Geometry: final body of the model. Coordinates: model frame, mm. A direction names the side the tool comes from. Coordinates: 2 decimals unless noted, no trailing zeros. Loops run counter-clockwise (first coordinate to the right, second up) from the corner with the lowest first, then second, coordinate; pieces in that order, holes last. Notation, with made-up numbers: (-7, 66.25) -> (48, 66.25) arc R23 cw to (48, 92.25) -> close; hole circle Ø8 at (-32, 89). An arc over 180 degrees is marked (long way). One line per item, written item: value. Start each with the question number.
Item 1: Contact query for flat-ended pins moving along their axis: pin 1 Ø5 at (x, y) = (-22, -31.5) entering from +Z; pin 2 Ø5 at (x, z) = (-63, 3.5) entering from -Y; pin 3 Ø11.5 at (x, z) = (-56.5, 30.5) entering from -Y; pin 4 Ø8.5 at (x, y) = (-47.5, -6.5) entering from +Z. Output: stop coordinate, or through.
Item 2: Mould query, pull axis X, two halves, no side actions, for faces 1 (the flat face through (0, -38, 24)), 2 (the flat face through (-11.313, -38, 29)), 3 (the flat face through (-91, -76.2, 24)). Classes: +X half, -X half, draft (parallel to the pull), parting line (faces both ways), or undercut.
Item 3: Ray query, probe 1 along X at (y, z) = (-60, 45.5); probe 2 along Y at (x, z) = (-90, 24.5); probe 3 along Y at (x, z) = (-21, 45). Return the intervals inside material, ascending. Write a range as from..to.
Item 4: Set-up query: faces 4 (the cylindrical face through (-10.787, -73.222, 43.681)), 5 (the flat face through (-51, -6, 23.301)), 6 (the flat face through (-53, -37, 9.625)), 7 (the flat face through (-51, -63.792, 5)). Return all of +Z, -Z, +X, -X, +Y, -Y with unobstructed straight access to the full face (end or side cutting, diameter ignored); none if empty.
Item 5: Section query D-D on y = -68. Return loops of the section in (x, z).
Item 6: Section query C-C on y = -44. Return loops of the section in (x, z).
Item 7: Section query A-A on z = 37. Return loops of the section in (x, y).
Item 8: Section query B-B on x = -60. Return loops of the section in (y, z).
from build123d import *

# Parameters (mm, degrees)
F0_W      = 101.346001029
F0_H      = 47.725263983
F1_DEPTH  = 76.2
F2_W      = 81.5831655636
F2_H      = 52.9085965827
F3_DEPTH  = 38.1
F4_W      = 58.673998341
F4_H      = 24.4241077453
F5_DEPTH  = 76.2
F6_W      = 58.673998341
F6_H      = 12.4078532577
F7_DEPTH  = 50.8
F8_R      = 3.5544652988
F9_DEPTH  = 127
F10_R     = 3.7666020305
F11_DEPTH = 127


with BuildPart() as f1:
    # F0 (on Front) → F1 (new body)
    with BuildSketch(Plane.XZ):
        with Locations((-50.6730005145, 23.8626319915)):
            Rectangle(F0_W, F0_H)
    extrude(amount=F1_DEPTH)

    # F2 (on face) → F3 (cut)
    with BuildSketch(Plane.XY.offset(47.725263983)):
        with Locations((-52.104968112, -37.337848451)):
            Rectangle(F2_W, F2_H)
    extrude(amount=-F3_DEPTH, mode=Mode.SUBTRACT)

    # F4 (on face) → F5 (cut)
    with BuildSketch(Plane.XZ.offset(76.2)):
        with Locations((-50.6128417328, 35.5132101104)):
            Rectangle(F4_W, F4_H)
    extrude(amount=-F5_DEPTH, mode=Mode.SUBTRACT)

    # F6 (on face) → F7 (cut)
    with BuildSketch(Plane.XY.offset(23.3011562377)):
        with Locations((-50.6128417328, -69.9960733712)):
            Rectangle(F6_W, F6_H)
    extrude(amount=-F7_DEPTH, mode=Mode.SUBTRACT)

    # F8 (on face) → F9 (cut)
    with BuildSketch(Plane(origin=(-101.346001029, 0, 0), x_dir=(0, -1, 0), z_dir=(-1, 0, 0))):
        with Locations((68.0850967765, 9.1249775141)):
            Circle(F8_R)
    extrude(amount=-F9_DEPTH, mode=Mode.SUBTRACT)

    # F10 (on face) → F11 (cut)
    with BuildSketch(Plane(origin=(-101.346001029, 0, 0), x_dir=(0, -1, 0), z_dir=(-1, 0, 0))):
        with Locations((69.6296393871, 42.5492078066)):
            Circle(F10_R)
    extrude(amount=-F11_DEPTH, mode=Mode.SUBTRACT)


solid = f1.part
Reply:
1. pin 1: stops at z = 9.63
1. pin 2: stops at y = -63.79
1. pin 3: passes through
1. pin 4: stops at z = 23.3
2. face 1: +X half
2. face 2: undercut
2. face 3: draft
3. probe 1: x = -101.35..-92.9, -11.31..0
3. probe 2: y = -76.2..-63.79, -10.88..0
3. probe 3: y = -76.2..-72.49, -66.77..-63.79, -10.88..0
4. face 4: +X, -X
4. face 5: +Z, +Y, -Y
4. face 6: +Z
4. face 7: +Z, -Z, -Y
5. outline: (-101.35, 0) -> (-79.95, 0) -> (-79.95, 5.57) -> (-101.35, 5.57) -> close; (-101.35, 12.68) -> (-79.95, 12.68) -> (-79.95, 39.15) -> (-101.35, 39.15) -> close; (-101.35, 45.95) -> (-79.95, 45.95) -> (-79.95, 47.73) -> (-101.35, 47.73) -> close; (-21.28, 0) -> (0, 0) -> (0, 5.57) -> (-21.28, 5.57) -> close; (-21.28, 12.68) -> (0, 12.68) -> (0, 39.15) -> (-21.28, 39.15) -> close; (-21.28, 45.95) -> (0, 45.95) -> (0, 47.73) -> (-21.28, 47.73) -> close
6. outline: (-101.35, 0) -> (0, 0) -> (0, 47.73) -> (-11.31, 47.73) -> (-11.31, 9.63) -> (-92.9, 9.63) -> (-92.9, 47.73) -> (-101.35, 47.73) -> close
7. outline: (-101.35, -76.2) -> (-79.95, -76.2) -> (-79.95, -63.79) -> (-92.9, -63.79) -> (-92.9, -10.88) -> (-79.95, -10.88) -> (-79.95, 0) -> (-101.35, 0) -> close; (-21.28, -76.2) -> (0, -76.2) -> (0, 0) -> (-21.28, 0) -> (-21.28, -10.88) -> (-11.31, -10.88) -> (-11.31, -63.79) -> (-21.28, -63.79) -> close
8. outline: (-63.79, 0) -> (0, 0) -> (0, 23.3) -> (-10.88, 23.3) -> (-10.88, 9.63) -> (-63.79, 9.63) -> close
